Here's how the part is built. I have some questions about the finished solid (model axes, mm). A direction names the side the tool comes from. Coordinates: 2 decimals unless noted, no trailing zeros. Write each loop counter-clockwise with the first axis right and the second up, starting at its lowest first coordinate (ties: lowest second). Pieces come first, ordered by that corner, then holes. Notation, with made-up numbers: (26.5, -37.5) -> (53.5, -37.5) arc R12 cw to (53.5, -18.5) -> close; hole circle Ø4 at (35, 19.5). An arc over 180 degrees is marked (long way). Use a Markdown table: item, result. Add a question column.
```python
from build123d import *

# Parameters (mm, degrees)
F0_W     = 49.266301
F0_H     = 47.738668
F1_DEPTH = 25.4
F2_W     = 17.185921
F2_H     = 17.185918
F3_DEPTH = 17.78
F4_R     = 9.270667
F5_DEPTH = 20.32
F6_R     = 9.183708
F7_DEPTH = 50.8


with BuildPart() as f1:
    # F0 (on Front) → F1 (new body)
    with BuildSketch(Plane.XZ):
        with Locations((4.010047, 0.572864)):
            Rectangle(F0_W, F0_H)
    extrude(amount=F1_DEPTH)

    # F2 (on face) → F3 (join)
    with BuildSketch(Plane.XZ.offset(25.4)):
        with Locations((14.894463, 11.648234)):
            Rectangle(F2_W, F2_H)
    extrude(amount=F3_DEPTH)

    # F4 (on face) → F5 (join)
    with BuildSketch(Plane.XZ.offset(25.4)):
        with Locations((-5.833408, -13.375082)):
            Circle(F4_R)
    extrude(amount=F5_DEPTH)

    # F6 (on face) → F7 (cut)
    with BuildSketch(Plane.YZ.offset(28.643198)):
        with Locations((-15.085418, 0)):
            Circle(F6_R)
    extrude(amount=-F7_DEPTH, mode=Mode.SUBTRACT)


solid = f1.part
```
Q1. Which directions (+Z, -Z, +X, -X, +Y, -Y) give clear straight access to the entire face, cutting with the end or side of a thin tool? Please do faces 1 (the flat face through (15, -34, 3.055)), 2 (the flat face through (23.487, -34, 12)), 3 (the flat face through (15, -34, 20.241)).
Q2. Will these pins go through, and if not, where does the flat tip stop? pin 1 (19 mm diameter, centred on x = 17, y = -32.5, fed in from -Z); pin 2 (11 mm diameter, centred on y = -15.09, z = 0, fed in from +X); pin 3 (13.5 mm diameter, centred on x = 15.5, y = -37.5, fed in from +Z); pin 4 (8 mm diameter, centred on y = -38.5, z = 6, fed in from +X).
Q3. Please list where these lines run through material, in increasing order: line 1 (Y direction, x = -10, z = 18); line 2 (Z direction, x = 9.5, y = -41.5); line 3 (Z direction, x = 25, y = -21.5).
Q4. Suppose I cut it at A-A, the plane z = 0. Write out the boundary of the cut face in (x, y).
Q5. Thinking about a two-plate mould opening in Z: for faces 4 (the cylindrical face through (4.355, -17.076, -8.965)), 5 (the flat face through (4, -13, 24.442)), 6 (the flat face through (-20.623, -7, -5)), which applies, released by +Z, released by -Z, zero draft, split by the parting line, or undercut?
Q6. Suppose I cut it at B-B, the plane y = -9. Write out the boundary of the cut face in (x, z), and give its area (3 significant figures).
Q7. Suppose I cut it at C-C, the plane x = 14. Write out the boundary of the cut face in (y, z).
Q8. Suppose I cut it at D-D, the plane x = 2.5. Write out the boundary of the cut face in (y, z).
Answer key:
| question | item | result |
|---|---|---|
| 1 | face 1 | -Z, +X, -X, -Y |
| 1 | face 2 | +Z, -Z, +X, -Y |
| 1 | face 3 | +Z, +X, -X, -Y |
| 2 | pin 1 | stops at z = -23.3 |
| 2 | pin 2 | passes through |
| 2 | pin 3 | stops at z = 20.24 |
| 2 | pin 4 | stops at x = 23.49 |
| 3 | line 1 | y = -25.4 to 0 |
| 3 | line 2 | z = 3.06 to 20.24 |
| 3 | line 3 | z = -23.3 to -6.57, 6.57 to 24.44 |
| 4 | outline | (-20.62, -25.4) -> (28.64, -25.4) -> (28.64, -24.27) -> (-20.62, -24.27) -> close; (-20.62, -5.9) -> (28.64, -5.9) -> (28.64, 0) -> (-20.62, 0) -> close |
| 5 | face 4 | undercut |
| 5 | face 5 | released by +Z |
| 5 | face 6 | zero draft |
| 6 | outline | (-20.62, -23.3) -> (28.64, -23.3) -> (28.64, -6.88) -> (-20.62, -6.88) -> close; (-20.62, 6.88) -> (28.64, 6.88) -> (28.64, 24.44) -> (-20.62, 24.44) -> close |
| 6 | area | 1,670 mm^2 |
| 7 | outline | (-43.18, 3.06) -> (-25.4, 3.06) -> (-25.4, -23.3) -> (0, -23.3) -> (0, 24.44) -> (-25.4, 24.44) -> (-25.4, 20.24) -> (-43.18, 20.24) -> close; hole circle Ø18.37 at (-15.09, 0) |
| 8 | outline | (-45.72, -17.44) -> (-25.4, -17.44) -> (-25.4, -23.3) -> (0, -23.3) -> (0, 24.44) -> (-25.4, 24.44) -> (-25.4, -9.31) -> (-45.72, -9.31) -> close; hole circle Ø18.37 at (-15.09, 0) |
